Autodesk Inventor part; units mm, degrees
ref_plane "Work Plane1" through (29, 0, 0) normal (0, -1, 0) x (1, 0, 0)
ref_plane "YZ Plane" through (0, 0, 0) normal (1, 0, 0) x (0, 1, 0)
ref_plane "XZ Plane" through (0, 0, 0) normal (0, 1, 0) x (-1, 0, 0)
sketch "Sketch1" plane through (0, 0, 0) normal (0, 0, 1) x (1, 0, 0)
  line L0 (-0.6, 0) -> (10, 0)
  line L1 (10, 0) -> (10, 2.5)
  line L2 (10, 2.5) -> (7, 2.5)
  line L3 (7, 2.5) -> (6.6932, 2.5)
  line L4 (6.6932, 2.5) -> (0, 2.5)
  line L5 (0, 2.5) -> (0, 4.75)
  line L6 (0, 4.75) -> (-2.6, 4.75)
  line L7 (-2.6, 4.75) -> (-2.6, 1.7321)
  line L8 (-2.6, 1.7321) -> (-1.6, 1.7321)
  line L9 (-1.6, 1.7321) -> (-0.6, 0)
  line L10 (-5.12, 0) -> (12.52, 0)
  line L11 (0, -0.95) -> (0, 5.7)
  line L12 (7, 2.5) -> (0, 2.5) construction
  dimension "d1" = 3
  dimension "d2" = 0.3068
  dimension "d3" = 2.6
  dimension "d4" = 1
  dimension "d5" = 60
  dimension "d6" = 5
  dimension "d7" = 5
  dimension "d8" = 3.4641
  dimension "d9" = 9.5
  dimension "d26" = 10
revolve "Body" add sketch "Sketch1" angle 360 about axis through (-0.6, 0, 0) along (1, 0, 0)
sketch "Sketch2" plane through (-2.6, 0, 0) normal (-1, 0, 0) x (0, 0, 1)
  circle A0 centre (0, 0) radius 1.7321
  line L0 (0, -6.65) -> (0, 6.65)
  line L1 (-6.65, 0) -> (6.65, 0)
  line L2 (1.7321, 0) -> (0.866, -1.5)
  line L3 (0.866, -1.5) -> (-0.866, -1.5)
  line L4 (-0.866, -1.5) -> (-1.7321, 0)
  line L5 (-1.7321, 0) -> (-0.866, 1.5)
  line L6 (-0.866, 1.5) -> (0.866, 1.5)
  line L7 (0.866, 1.5) -> (1.7321, 0)
extrude "Slot" add sketch "Sketch2" against normal up to next contours L7 A0 | A0 L2 | L6 L0 A0 | A0 L0 L3 | L0 L6 A0 | A0 L3 L0 | L4 A0 | A0 L5
fillet "Fillet1" radius 1.2 1 edges at (-2.6, -4.75, 0)
chamfer "Chamfer1" distance 0.3067 distance2 0.3067 1 edges at (10, -2.5, 0) measured on face at (10, -0.7741, -0.6858)
ref_plane "Work Plane1" through (29, 0, 0) normal (0, -1, 0) x (1, 0, 0)
fillet "Fillet2" radius 0.1 1 edges at (0, -2.5, 0)
thread "Thread2"
equation "\"d15\" = -0.5 * SPD + 0.5 * GD"
equation "\"d16\" = GUL"
equation "\"GD\" = NND"
equation "\"NLG\" = 6"
equation "\"GEL\" = 4.5"
equation "\"KOD\" = 5.7"
equation "\"KOH\" = 1.65"
equation "\"INTI\" = 1.04"
equation "\"GAL\" = 0.61345 * PTC"
equation "\"GUL\" = 0.61345 * PTC"
equation "\"BDM\" = NND"
equation "\"SW\" = 2"
equation "\"RR\" = 1.45"
equation "\"SPD\" = NND - 1.2269 * PTC"
equation "\"R\" = 0.3"
equation "\"TOA\" = 30deg"
equation "\"GD1\" = THREADDIA - 1.2269 * PTC"
equation "\"THREADDIA\" = 3"
equation "\"PTC\" = 0.5"
equation "\"NND\" = 3"
equation "\"KOH1\" = 0.2"
equation "\"E0\" = 2.303"
properties part number "M5x10 Bolt" material "Stainless Steel"
Can you work these out from the model? Positions are in its coordinate system, mm. A direction names the side the tool comes from. Coordinates: 2 decimals unless noted, no trailing zeros. Order: outer loops, then holes, each group sorted by start corner. A loop starts at its lowest first (then second) coordinate and runs counter-clockwise, first axis right, second up.
1. Thinking about a two-plate mould opening in Y: for faces 4 (the face through (4.83, -0.54, 2.44)), 5 (the face through (-2.6, -2, 0)), 6 (the face through (-2, -1.5, 0)), which applies, +Y half, -Y half, draft (parallel to the pull), parting line (faces both ways), or undercut?
2. I need wall thicknesses on line 1 (X direction, y = -3, z = -1.5); line 2 (X direction, y = 2.75, z = 3.5); line 3 (Z direction, x = 7.5, y = -2). Which ranges of each line are inside material? Lowest first, please.
3. I'm going to push flat-ended pins straight in: pin 1 (1 mm diameter, centred on y = -2, z = -1, fed in from +X); pin 2 (5 mm diameter, centred on x = 1, z = 2.5, fed in from +Y); pin 3 (0.6 mm diameter, centred on x = -2, z = 0.5, fed in from -Y). Where does each tip first touch, or does it pass through?
4. If we section it at A-A (x = 5): Please give me the cut outline in (y, z).
5. If we section it at B-B (x = -1.25): Please give me the cut outline in (y, z), then the cut area to 3 significant figures.
6. For faces 1 (the face through (0, 2, -2)), 2 (the face through (10, 0, 0)), 3 (the face through (-2.041, -0.761, -1.293)), which set-ups out of +Z, -Z, +X, -X, +Y, -Y let a thin tool reach every point of the face, with its end or its side?
Entries:
1. face 4: parting line
1. face 5: draft
1. face 6: undercut
2. line 1: x = -2.6 to 0
2. line 2: x = -2.19 to 0
2. line 3: z = -1.5 to 1.5
3. pin 1: stops at x = 10
3. pin 2: stops at y = 4.75
3. pin 3: stops at y = -4.69
4. outline: circle Ø5 at (0, 0)
5. outline: circle Ø9.5 at (0, 0); hole circle Ø2.25 at (0, 0)
5. area: 66.9 mm2
6. face 1: +X
6. face 2: +Z, -Z, +X, +Y, -Y
6. face 3: -X
